The listing builds one solid part. Answer for the finished solid, in the listing's coordinates (mm). A direction names the side the tool comes from. Coordinates: 2 decimals unless noted, no trailing zeros. Order: outer loops, then holes, each group sorted by start corner. A loop starts at its lowest first (then second) coordinate and runs counter-clockwise, first axis right, second up. Notation, with made-up numbers: (80, -26) - (114, -26) arc R27 ccw to (114, 7) - close; hole circle Ø10 at (19, -39.75). An arc over 180 degrees is marked (long way). One line per item, written item: value. Start each with the question number.
```python
from build123d import *

# Parameters (mm, degrees)
F1_DEPTH = 12
F3_DEPTH = 10
F4_W     = 5
F4_H     = 5
F4_H_2   = 3
F5_DEPTH = 170
F6_W     = 5
F6_H     = 8
F7_DEPTH = 12.7
F9_DEPTH = 25


with BuildPart() as f1:
    # F0 (on Front) → F1 (new body)
    with BuildSketch(Plane.XZ):
        with BuildLine():
            Line((0, 8), (0, 6.5))
            ThreePointArc((0, 6.5), (1.2747548784, 6.373774392), (2.5, 6))
            Line((2.5, 6), (2.5, 7.5993420768))
            ThreePointArc((2.5, 7.5993420768), (1.2659509046, 7.8992004853), (0, 8))
        make_face()
        with BuildLine():
            ThreePointArc((-2.5, 6), (-1.2747548784, 6.373774392), (0, 6.5))
            Line((0, 6.5), (0, 8))
            ThreePointArc((0, 8), (-1.2659509046, 7.8992004853), (-2.5, 7.5993420768))
            Line((-2.5, 7.5993420768), (-2.5, 6))
        make_face()
        with BuildLine():
            Line((2.5, 7.5993420768), (2.5, 6))
            ThreePointArc((2.5, 6), (5.4083269132, 3.6055512755), (6.5, 0))
            ThreePointArc((6.5, 0), (-3.6055512755, -5.4083269132), (-2.5, 6))
            Line((-2.5, 6), (-2.5, 7.5993420768))
            ThreePointArc((-2.5, 7.5993420768), (-4.6904157598, -6.4807406984), (8, 0))
            ThreePointArc((8, 0), (6.4807406984, 4.6904157598), (2.5, 7.5993420768))
        make_face()
        with BuildLine():
            ThreePointArc((-2.5, 13.8348486101), (-1.2611625184, 13.5840842664), (0, 13.5))
            Line((0, 13.5), (0, 14.832704328))
            Line((0, 14.832704328), (-2.5, 14.832704328))
            Line((-2.5, 14.832704328), (-2.5, 13.8348486101))
        make_face()
        with BuildLine():
            Line((0, 14.832704328), (0, 13.5))
            ThreePointArc((0, 13.5), (1.2611625184, 13.5840842664), (2.5, 13.8348486101))
            Line((2.5, 13.8348486101), (2.5, 14.832704328))
            Line((2.5, 14.832704328), (0, 14.832704328))
        make_face()
        with BuildLine():
            Line((-2.5, 14.832704328), (0, 14.832704328))
            Line((0, 14.832704328), (2.5, 14.832704328))
            Line((2.5, 14.832704328), (2.5, 13.8348486101))
            ThreePointArc((2.5, 13.8348486101), (7.5498344353, 17.2337187027), (9.5, 23))
            ThreePointArc((9.5, 23), (-5.7662812973, 30.5498344353), (-2.5, 13.8348486101))
            Line((-2.5, 13.8348486101), (-2.5, 14.832704328))
        make_face()
        with BuildLine():
            ThreePointArc((7.5, 23), (5.3033008589, 17.6966991411), (0, 15.5))
            ThreePointArc((0, 15.5), (-5.3033008589, 28.3033008589), (7.5, 23))
        make_face(mode=Mode.SUBTRACT)
        with BuildLine():
            Line((0, 13.5), (0, 8))
            ThreePointArc((0, 8), (1.2659509046, 7.8992004853), (2.5, 7.5993420768))
            Line((2.5, 7.5993420768), (2.5, 13.8348486101))
            ThreePointArc((2.5, 13.8348486101), (1.2611625184, 13.5840842664), (0, 13.5))
        make_face()
        with BuildLine():
            ThreePointArc((-2.5, 7.5993420768), (-1.2659509046, 7.8992004853), (0, 8))
            Line((0, 8), (0, 13.5))
            ThreePointArc((0, 13.5), (-1.2611625184, 13.5840842664), (-2.5, 13.8348486101))
            Line((-2.5, 13.8348486101), (-2.5, 7.5993420768))
        make_face()
    extrude(amount=F1_DEPTH)

    # F2 (on Front) → F3 (join)
    with BuildSketch(Plane.XZ):
        Polygon((5, -6.5), (0, -6.5), (-5, -6.5), (-5, -29.5), (-10, -29.5), (-10, -51), (10, -51), (10, -29.5), (5, -29.5), align=None)
    extrude(amount=F3_DEPTH)

    # F4 (on Front) → F5 (join)
    with BuildSketch(Plane.XZ):
        with Locations((7.5, -48.5)):
            Rectangle(F4_W, F4_H)
        with Locations((7.5, -34.4996317649)):
            Rectangle(F4_W, F4_H_2)
        with Locations((-7.5, -34.4996317649)):
            Rectangle(F4_W, F4_H_2)
        Polygon((-5, -46), (-5, -45.9992635297), (-10, -45.9992635297), (-10, -51), (-5, -51), align=None)
    extrude(amount=-F5_DEPTH)

    # F6 (on face) → F7 (join)
    with BuildSketch(Plane(origin=(0, 0, -35.9996317649), x_dir=(1, 0, 0), z_dir=(0, 0, -1))):
        with Locations((-7.5, -166)):
            Rectangle(F6_W, F6_H)
        with Locations((7.5, -166)):
            Rectangle(F6_W, F6_H)
    extrude(amount=F7_DEPTH)

    # F8 (on face) → F9 (cut)
    with BuildSketch(Plane(origin=(-10, 0, 0), x_dir=(0, -1, 0), z_dir=(-1, 0, 0))):
        with BuildLine():
            Line((-162, -35.9996317649), (-161.9570914715, -35.9996317649))
            ThreePointArc((-161.9570914715, -35.9996317649), (-167, -40.9994476473), (-161.9570914715, -45.9992635297))
            Line((-161.9570914715, -45.9992635297), (-162, -45.9992635297))
            Line((-162, -45.9992635297), (-162, -35.9996317649))
        make_face()
        with BuildLine():
            ThreePointArc((-161.9570914715, -45.9992635297), (-158.4493280465, -44.51977841), (-157, -40.9994476473))
            ThreePointArc((-157, -40.9994476473), (-158.4493280465, -37.4791168846), (-161.9570914715, -35.9996317649))
            Line((-161.9570914715, -35.9996317649), (-162, -35.9996317649))
            Line((-162, -35.9996317649), (-162, -45.9992635297))
            Line((-162, -45.9992635297), (-161.9570914715, -45.9992635297))
        make_face()
    extrude(amount=-F9_DEPTH, mode=Mode.SUBTRACT)


solid = f1.part
```
(1) The part is cut by section B-B on z = -40.5. Determine the outline of the cut face in (x, y) (3 decimals), plus the area to 3 significant figures.
(2) Flat-ended cylindrical pins translate along their axes: pin 1 Ø5 at (y, z) = (107.5, -41) entering from +X (3 decimals); pin 2 Ø4 at (x, z) = (-3.5, 3.5) entering from +Y; pin 3 Ø10 at (x, z) = (-2, -28) entering from -Y; pin 4 Ø4 at (x, z) = (3.5, -32.5) entering from +Y. Find the tip coordinate at first contact, or state that the pin passes through.
(3) Consider probe 1 along X at (y, z) = (-3.5, 23); probe 2 along Z at (x, y) = (-7.75, 150.5); probe 3 along Y at (x, z) = (3.75, -20.5). Determine where each line is inside the solid, lowest interval first.
(4) For faces 1 (the face through (-7, -5, -29.5)), 2 (the face through (-8, 84, -33)), 3 (the face through (-7, 80, -45.999)), 4 (the face through (-5, 86, -48)), determine the directions among +Z, -Z, +X, -X, +Y, -Y from which every point of the face is accessible in a straight line to the end or side of a thin tool.
(5) For a pull along X with two mould halves and no side action, classify faces 5 (the face through (7, 84, -33)), 6 (the face through (10, 78.7, -35.6)), 7 (the face through (5, 84, -48)) as pulls with the +X half, pulls with the -X half, needs draft (parallel to the pull), parting line crosses it, or undercut.
(6) The part is cut by section C-C on z = -2. Determine the outline of the cut face in (x, y), plus the area to 3 significant figures.
(7) The part is cut by section A-A on y = 88.5. Determine the outline of the cut face in (x, z).
Completed:
1. outline: (-10, -10) - (10, -10) - (10, 0) - (-10, 0) - close; (-10, 166.975) - (-5, 166.975) - (-5, 170) - (-10, 170) - close; (5, 166.975) - (10, 166.975) - (10, 170) - (5, 170) - close
1. area: 230 mm2
2. pin 1: passes through
2. pin 2: stops at y = 0
2. pin 3: stops at y = -10
2. pin 4: stops at y = 170
3. probe 1: x = -9.5 to -7.5, 7.5 to 9.5
3. probe 2: z = -51 to -46, -36 to -33
3. probe 3: y = -10 to 0
4. face 1: -X, +Y, -Y
4. face 2: +Z, +X, -X, +Y
4. face 3: +X, -X
4. face 4: +Z, -Z, +Y
5. face 5: needs draft
5. face 6: pulls with the +X half
5. face 7: undercut
6. outline: (-7.75, -12) - (-6.18, -12) - (-6.18, 0) - (-7.75, 0) - close; (6.18, -12) - (7.75, -12) - (7.75, 0) - (6.18, 0) - close
6. area: 37.5 mm2
7. outline: (-10, -51) - (-5, -51) - (-5, -46) - (-10, -46) - close; (-10, -36) - (-5, -36) - (-5, -33) - (-10, -33) - close; (5, -51) - (10, -51) - (10, -46) - (5, -46) - close; (5, -36) - (10, -36) - (10, -33) - (5, -33) - close
